```python
from build123d import *

# Parameters (mm, degrees)
F0_R     = 49.2125
F0_R_2   = 5.159375
F1_DEPTH = 6.35
F3_D     = 8.7376


with BuildPart() as f1:
    # F0 (on Front) → F1 (new body)
    with BuildSketch(Plane.XZ):
        Circle(F0_R)
        with Locations((-28.0633, -28.0633)):
            Circle(F0_R_2, mode=Mode.SUBTRACT)
        with Locations((28.0633, -28.0633)):
            Circle(F0_R_2, mode=Mode.SUBTRACT)
        with Locations((-28.0633, 28.0633)):
            Circle(F0_R_2, mode=Mode.SUBTRACT)
        with Locations((28.0633, 28.0633)):
            Circle(F0_R_2, mode=Mode.SUBTRACT)
    extrude(amount=F1_DEPTH)

    # F3 (through all)
    with Locations(Plane.XZ.offset(6.35)):
        with Locations((0, 35.245303), (34.716293, 6.083617), (0, -35.245303), (-34.716293, -6.083617)):
            Hole(F3_D / 2)


solid = f1.part
```
CAD build for the part. Positions are in the model's coordinates, mm. Coordinates: 2 decimals unless noted, no trailing zeros. Order: outer loops, then holes, each group sorted by start corner. A loop starts at its lowest first (then second) coordinate and runs counter-clockwise, first axis right, second up. Notation, with made-up numbers: (68.25, -22.5) -> (125.25, -22.5) arc R20 ccw to (125.25, 0.5) -> close; hole circle Ø4 at (-4.5, -32.75). An arc over 180 degrees is marked (long way). Use one line per item in the form item = value. Start each with the question number.
1) Band-saw the part on C-C on y = -3.5. State how many separate pieces and enclosed holes the cut face has, then the cut area to 3 significant figures.
2) Drill centre lines: L1, parallel to Z at x = -1, y = -2.25; L2, parallel to Z at x = 1.5, y = -3.75; L3, parallel to X at y = -5.5, z = -37. Where is each one in solid material? Low to high. Write a range as [from, to].
3) Band-saw the part on D-D on x = 10. Give the cut face in (y, z), then the cut area to 3 significant figures.
4) Pull direction X, two halves, no side cores. Call faces 1 (the cylindrical face through (46.94, -3.13, 14.78)), 2 (the flat face through (-1, 0, 1)), 3 (the cylindrical face through (-2.02, -3.13, 31.37)): +X half, -X half, draft (parallel to the pull), parting line (faces both ways), or undercut.
5) Band-saw the part on A-A on x = 0. Give the cut face in (y, z), then the cut area to 3 significant figures.
6) Drop flat-ended pins along their axis: pin 1 (3 mm diameter, centred on x = -37.5, y = -5.5, fed in from -Z); pin 2 (10 mm diameter, centred on x = 0, z = 35.25, fed in from -Y); pin 3 (2 mm diameter, centred on x = -0.5, y = -3.5, fed in from +Z). Give the stop position or say it passes through.
7) Band-saw the part on B-B on z = -38. Give the cut face in (x, y).
Entries:
q1.separate_pieces = 1
q1.enclosed_holes = 8
q1.area = 7,030 mm2
q2.L1 = [-49.2, -39.5], [-30.99, 30.99], [39.5, 49.2]
q2.L2 = [-49.19, -39.35], [-31.14, 31.14], [39.35, 49.19]
q2.L3 = [-32.45, -4], [4, 32.45]
q3.outline = (-6.35, -48.19) -> (0, -48.19) -> (0, 48.19) -> (-6.35, 48.19) -> close
q3.area = 612 mm2
q4.face_1 = parting line
q4.face_2 = draft
q4.face_3 = undercut
q5.outline = (-6.35, -49.21) -> (0, -49.21) -> (0, -39.61) -> (-6.35, -39.61) -> close; (-6.35, -30.88) -> (0, -30.88) -> (0, 30.88) -> (-6.35, 30.88) -> close; (-6.35, 39.61) -> (0, 39.61) -> (0, 49.21) -> (-6.35, 49.21) -> close
q5.area = 514 mm2
q6.pin_1 = -33.55
q6.pin_2 = -6.35
q6.pin_3 = 49.21
q7.outline = (-31.27, -6.35) -> (-3.39, -6.35) -> (-3.39, 0) -> (-31.27, 0) -> close; (3.39, -6.35) -> (31.27, -6.35) -> (31.27, 0) -> (3.39, 0) -> close
